```python
from build123d import *

# Parameters (mm, degrees)
SKETCH1_W            = 45.45
SKETCH1_H            = 20
BOSS_EXTRUDE1_DEPTH  = 8
SKETCH2_W            = 37.45
SKETCH2_H            = 5.9
BOSS_EXTRUDE2_DEPTH  = 0.8
M3_CLEARANCE_HOLE1_D = 3.4


with BuildPart() as part:
    # Sketch1 → Boss-Extrude1 (new body)
    with BuildSketch(Plane(origin=(0, 0, 0), x_dir=(1, 0, 0), z_dir=(0, 1, 0))):
        with Locations((7.654765617, -1.92370193)):
            Rectangle(SKETCH1_W, SKETCH1_H)
    extrude(amount=BOSS_EXTRUDE1_DEPTH)

    # Sketch2 → Boss-Extrude2 (add)
    with BuildSketch(Plane(origin=(0, 8, 0), x_dir=(1, 0, 0), z_dir=(0, 1, 0))):
        with Locations((7.654765617, -1.92370193)):
            Rectangle(SKETCH2_W, SKETCH2_H)
    extrude(amount=BOSS_EXTRUDE2_DEPTH)

    # M3 Clearance Hole1 (through all)
    with Locations(Plane(origin=(0, 0, 0), x_dir=(-1, 0, 0), z_dir=(0, -1, 0))):
        with Locations((-20.379765617, -1.92370193), (5.070234383, -1.92370193)):
            Hole(M3_CLEARANCE_HOLE1_D / 2)


solid = part.part
```
CAD build for the part. Positions are in the model's coordinates, mm. A direction names the side the tool comes from. Give positions to 0.01 mm unless a question says otherwise; leave off trailing zeros. Order: outer loops, then holes, each group sorted by start corner. A loop starts at its lowest first (then second) coordinate and runs counter-clockwise, first axis right, second up.
(1) Flat gauge pins, fed straight in: pin 1 (0.6 mm diameter, centred on y = 8.5, z = 1.5, fed in from +X); pin 2 (0.6 mm diameter, centred on y = 8.5, z = 1, fed in from -X); pin 3 (2 mm diameter, centred on x = 20.38, z = 1.92, fed in from -Y). Where does each tip first touch, or does it go through?
(2) Mould opens along X. For faces 1 (the flat face through (26.38, 8.4, 2)), 2 (the flat face through (-11.07, 8.4, 2)), 3 (the cylindrical face through (-5.439, 4.462, 3.583)) say: released by +X, released by -X, zero draft, split by the parting line, or undercut.
(3) Saw through at D-D, the plane z = 1.5. Give the cut face in (x, y).
(4) Saw through at B-B, the plane z = 4.25. Give the cut face in (x, y), then the cut area to 3 significant figures.
(5) Saw through at C-C, the plane y = 2. Give the cut face in (x, z).
(6) Tool access for faces 4 (the flat face through (30.38, 4, 2)), 5 (the flat face through (7.4, 8.4, 4.874)), 6 (the flat face through (7.4, 8.4, -1.026)): list every direction of +Z, -Z, +X, -X, +Y, -Y with a clear straight run to the whole face (end or side of a thin tool).
(7) Saw through at A-A, the plane x = 6. Give the cut face in (y, z).
(8) Drill centre lines: L1, parallel to X at y = 4.75, z = 2.75; L2, parallel to Z at x = 20.5, y = 1; L3, parallel to Y at x = -7, z = 6.5. Where is each one in solid material? Low to high.
Results found:
1. pin 1: stops at x = 26.38
1. pin 2: stops at x = -11.07
1. pin 3: passes through
2. face 1: released by +X
2. face 2: released by -X
2. face 3: undercut
3. outline: (-15.07, 0) - (-6.72, 0) - (-6.72, 8.8) - (-11.07, 8.8) - (-11.07, 8) - (-15.07, 8) - close; (-3.42, 0) - (18.73, 0) - (18.73, 8.8) - (-3.42, 8.8) - close; (22.03, 0) - (30.38, 0) - (30.38, 8) - (26.38, 8) - (26.38, 8.8) - (22.03, 8.8) - close
4. outline: (-15.07, 0) - (30.38, 0) - (30.38, 8) - (26.38, 8) - (26.38, 8.8) - (-11.07, 8.8) - (-11.07, 8) - (-15.07, 8) - close
4. area: 394 mm2
5. outline: (-15.07, -8.08) - (30.38, -8.08) - (30.38, 11.92) - (-15.07, 11.92) - close; hole circle Ø3.4 at (-5.07, 1.92); hole circle Ø3.4 at (20.38, 1.92)
6. face 4: +Z, -Z, +X, +Y, -Y
6. face 5: +Z, +X, -X, +Y
6. face 6: -Z, +X, -X, +Y
7. outline: (0, -8.08) - (8, -8.08) - (8, -1.03) - (8.8, -1.03) - (8.8, 4.87) - (8, 4.87) - (8, 11.92) - (0, 11.92) - close
8. L1: x = -15.07 to -6.56, -3.58 to 18.89, 21.87 to 30.38
8. L2: z = -8.08 to 0.23, 3.62 to 11.92
8. L3: y = 0 to 8
